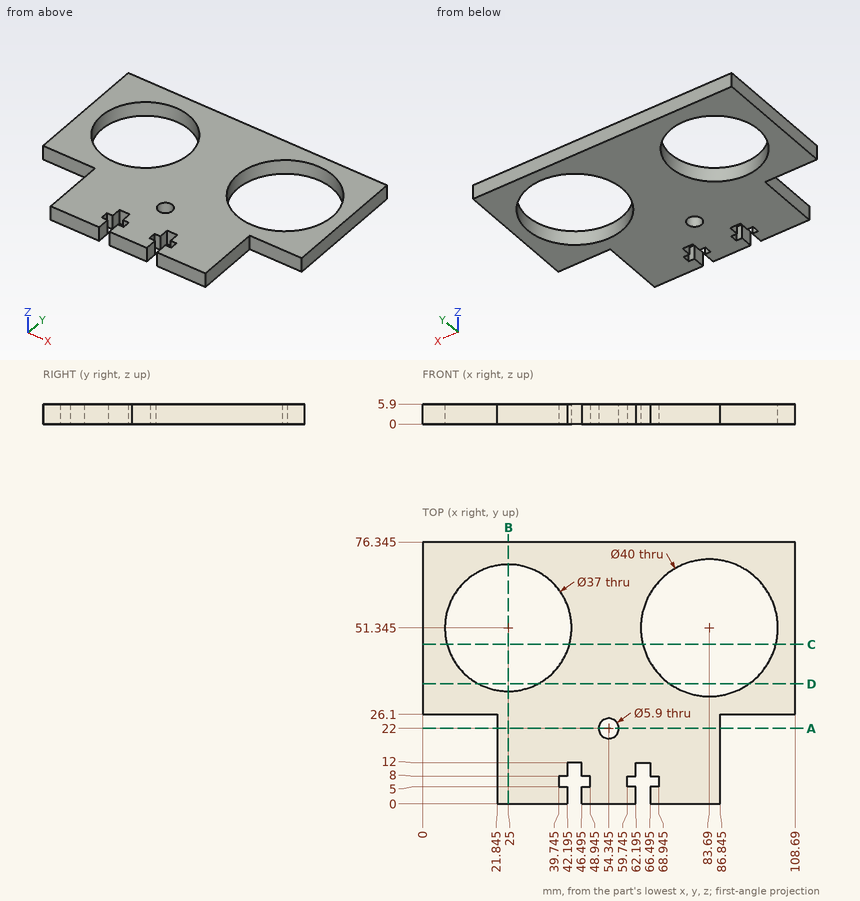
Could you check a few things on this drawing? It's one solid part, dimensions in mm from its lowest x, y, z. Give positions to 0.01 mm unless a question says otherwise; leave off trailing zeros. Order: outer loops, then holes, each group sorted by start corner. A loop starts at its lowest first (then second) coordinate and runs counter-clockwise, first axis right, second up. Notation, with made-up numbers: (79.5, 68.25) -> (87.5, 68.25) arc R12 ccw to (87.5, 85.25) -> close; hole circle Ø3 at (-19, -23.75). An arc over 180 degrees is marked (long way). Answer in a Markdown table with one row per item. Add a question column.
Item 1: I'm going to push flat-ended pins straight in: P1, Ø2.5, axis at y = 3.5, z = 1.5, coming from the -X side (3 decimals); P2, Ø1, axis at x = 44.5, y = 8.5, coming from the +Z side; P3, Ø2.5, axis at y = 2, z = 3.5, coming from the +X side (3 decimals); P4, Ø2, axis at x = 65, z = 2.5, coming from the -Y side. Where does each tip first touch, or does it pass through?
Item 2: Imagine slicing it at D-D (y = 35). List the corners of the cut face in (x, z) for me.
Item 3: Imagine slicing it at B-B (x = 25). List the corners of the cut face in (y, z) for me (3 decimals), and give its area (3 significant figures).
Item 4: Please list where these lines run through material, in increasing order: probe 1 along X at (y, z) = (8.5, 1.1) (3 decimals); probe 2 along X at (y, z) = (47.5, 2.7); probe 3 along X at (y, z) = (12.5, 4.65) (3 decimals).
Item 5: Imagine slicing it at A-A (y = 22). List the corners of the cut face in (x, z) for me (3 decimals).
Item 6: Imagine slicing it at C-C (y = 46.5). List the corners of the cut face in (x, z) for me.
Result:
| question | item | result |
|---|---|---|
| 1 | P1 | x = 21.845 |
| 1 | P2 | through |
| 1 | P3 | x = 86.845 |
| 1 | P4 | y = 12 |
| 2 | outline | (0, 0) -> (16.33, 0) -> (16.33, 5.9) -> (0, 5.9) -> close; (33.67, 0) -> (72.16, 0) -> (72.16, 5.9) -> (33.67, 5.9) -> close; (95.22, 0) -> (108.69, 0) -> (108.69, 5.9) -> (95.22, 5.9) -> close |
| 3 | outline | (0, 0) -> (32.845, 0) -> (32.845, 5.9) -> (0, 5.9) -> close; (69.845, 0) -> (76.345, 0) -> (76.345, 5.9) -> (69.845, 5.9) -> close |
| 3 | area | 232 mm2 |
| 4 | probe 1 | 21.845 to 42.195, 46.495 to 62.195, 66.495 to 86.845 |
| 4 | probe 2 | 0 to 6.9, 43.1 to 64.06, 103.32 to 108.69 |
| 4 | probe 3 | 21.845 to 86.845 |
| 5 | outline | (21.845, 0) -> (51.395, 0) -> (51.395, 5.9) -> (21.845, 5.9) -> close; (57.295, 0) -> (86.845, 0) -> (86.845, 5.9) -> (57.295, 5.9) -> close |
| 6 | outline | (0, 0) -> (7.15, 0) -> (7.15, 5.9) -> (0, 5.9) -> close; (42.85, 0) -> (64.29, 0) -> (64.29, 5.9) -> (42.85, 5.9) -> close; (103.09, 0) -> (108.69, 0) -> (108.69, 5.9) -> (103.09, 5.9) -> close |
